from build123d import *

# Parameters (mm, degrees)
SKETCH1_W                                           = 177.8
SKETCH1_H                                           = 150
BOSS_EXTRUDE1_DEPTH                                 = 41.6
SKETCH2_R                                           = 3.683
CUT_EXTRUDE1_DEPTH                                  = 42.6
CUT_EXTRUDE2_DEPTH                                  = 31.6
CBORE_FOR_M4_HEX_SOCKET_HEAD_CAP_SCREW1_D           = 4.5
CBORE_FOR_M4_HEX_SOCKET_HEAD_CAP_SCREW1_CBORE_D     = 8
CBORE_FOR_M4_HEX_SOCKET_HEAD_CAP_SCREW1_CBORE_DEPTH = 32.6
SKETCH9_W                                           = 177.8
SKETCH9_H                                           = 99.2
CUT_EXTRUDE4_DEPTH                                  = 1


with BuildPart() as part:
    # Sketch1 → Boss-Extrude1 (new body)
    with BuildSketch(Plane(origin=(0, 0, 0), x_dir=(1, 0, 0), z_dir=(0, 1, 0))):
        Rectangle(SKETCH1_W, SKETCH1_H)
    extrude(amount=BOSS_EXTRUDE1_DEPTH)

    # Sketch2 → Cut-Extrude1 (cut, through all)
    with BuildSketch(Plane(origin=(0, 41.6, 0), x_dir=(1, 0, 0), z_dir=(0, 1, 0))):
        with Locations(Location((63.5, -63.5, 0), (0, 0, 270))):  # turned: the seam where the file's is
            Circle(SKETCH2_R)
        with Locations(Location((-63.5, -63.5, 0), (0, 0, 270))):  # turned: the seam where the file's is
            Circle(SKETCH2_R)
    cut_extrude1 = extrude(amount=-CUT_EXTRUDE1_DEPTH, mode=Mode.SUBTRACT)

    # Sketch3 → Cut-Extrude2 (cut)
    with BuildSketch(Plane(origin=(0, 41.6, 0), x_dir=(1, 0, 0), z_dir=(0, 1, 0))):
        with BuildLine():
            Line((-74.93, -63.5), (-74.93, -75))
            Line((-74.93, -75), (-52.07, -75))
            Line((-52.07, -75), (-52.07, -63.5))
            ThreePointArc((-52.07, -63.5), (-63.5, -52.07), (-74.93, -63.5))
        make_face()
        with BuildLine():
            Line((52.07, -63.5), (52.07, -75))
            Line((52.07, -75), (74.93, -75))
            Line((74.93, -75), (74.93, -63.5))
            ThreePointArc((74.93, -63.5), (63.5, -52.07), (52.07, -63.5))
        make_face()
    cut_extrude2 = extrude(amount=-CUT_EXTRUDE2_DEPTH, mode=Mode.SUBTRACT)

    # Mirror1: Cut-Extrude1, Cut-Extrude2 across plane
    add(cut_extrude1.mirror(Plane(origin=(0, 0, 0), x_dir=(1, 0, 0), z_dir=(0, 0, -1))), mode=Mode.SUBTRACT)
    add(cut_extrude2.mirror(Plane(origin=(0, 0, 0), x_dir=(1, 0, 0), z_dir=(0, 0, -1))), mode=Mode.SUBTRACT)

    # CBORE for M4 Hex Socket Head Cap Screw1 (through all)
    with Locations(Plane.XZ):
        with Locations((68.9, 0), (-35.089800026, 50), (-35.089800026, -50)):
            CounterBoreHole(CBORE_FOR_M4_HEX_SOCKET_HEAD_CAP_SCREW1_D / 2, CBORE_FOR_M4_HEX_SOCKET_HEAD_CAP_SCREW1_CBORE_D / 2, CBORE_FOR_M4_HEX_SOCKET_HEAD_CAP_SCREW1_CBORE_DEPTH)

    # Sketch9 → Cut-Extrude4 (cut)
    with BuildSketch(Plane.XZ):
        Rectangle(SKETCH9_W, SKETCH9_H)
    extrude(amount=-CUT_EXTRUDE4_DEPTH, mode=Mode.SUBTRACT)


solid = part.part
Can you work these out from the model? Positions are in its coordinate system, mm. A direction names the side the tool comes from. Coordinates: 2 decimals unless noted, no trailing zeros. Loops run counter-clockwise (first coordinate to the right, second up) from the corner with the lowest first, then second, coordinate; pieces in that order, holes last. Notation, with made-up numbers: (88, 69.5) - (104, 69.5) arc R10 ccw to (104, 87.5) - close; hole circle Ø8 at (9, 62). An arc over 180 degrees is marked (long way). Put each result on its own line as item: value. Start each with the question number.
Item 1: Suppose I cut it at A-A (z = 0). Please give me the cut outline in (x, y).
Item 2: If we mould it in two halves opening along Z, with no side actions, what happens to faces 6 (the face through (72.595, 16.579, -1.532)), 7 (the face through (67.15, 5.07, -63.02)), 8 (the face through (63.751, 26.021, 52.073)), 9 (the face through (-52.07, 26, 69))? For each: +Z half, -Z half, draft (parallel to the pull), parting line (faces both ways), or undercut.
Item 3: Which directions (+Z, -Z, +X, -X, +Y, -Y) give clear straight access to the entire face, cutting with the end or side of a thin tool? Please do faces 1 (the face through (-33, 32.6, -52)), 2 (the face through (-59.85, 5.07, -63.02)), 3 (the face through (52.07, 26, -69)), 4 (the face through (52.07, 26, 69)), 5 (the face through (-88.9, 21, 1)).
Item 4: If I drill on line 1 along X through (y, z) = (2.5, -63.5); line 2 along X through (y, z) = (32.5, -59); line 3 along Y through (x, z) = (69, 67.5), over which ranges is the centre line in solid material (lowest first)?
Item 5: Suppose I cut it at B-B (y = 16). Please give me the cut outline in (x, z).
Item 6: Suppose I cut it at C-C (z = 40). Please give me the cut outline in (x, y).
Item 7: For pin 1 (6.5 mm diameter, centred on x = -63.5, z = -63.5, fed in from +Y); pin 2 (4 mm diameter, centred on x = -69.5, z = -35, fed in from -Y); pin 3 (7 mm diameter, centred on x = -35.09, z = 50, fed in from -Y), each with a flat end and sliding along its axis, tell me the tip position at first contact or that it passes through.
Here are the results:
1. outline: (-88.9, 1) - (64.9, 1) - (64.9, 32.6) - (66.65, 32.6) - (66.65, 41.6) - (-88.9, 41.6) - close; (71.15, 32.6) - (72.9, 32.6) - (72.9, 1) - (88.9, 1) - (88.9, 41.6) - (71.15, 41.6) - close
2. face 6: undercut
2. face 7: undercut
2. face 8: +Z half
2. face 9: draft
3. face 1: -Y
3. face 2: +Y, -Y
3. face 3: -Z, +Y
3. face 4: +Z, +Y
3. face 5: +Z, -Z, -X, +Y, -Y
4. line 1: -88.9 to -67.18, -59.82 to 59.82, 67.18 to 88.9
4. line 2: -88.9 to -74.01, -52.99 to 52.99, 74.01 to 88.9
4. line 3: 0 to 10
5. outline: (-88.9, -75) - (-74.93, -75) - (-74.93, -63.5) arc R11.43 cw to (-52.07, -63.5) - (-52.07, -75) - (52.07, -75) - (52.07, -63.5) arc R11.43 cw to (74.93, -63.5) - (74.93, -75) - (88.9, -75) - (88.9, 75) - (74.93, 75) - (74.93, 63.5) arc R11.43 cw to (52.07, 63.5) - (52.07, 75) - (-52.07, 75) - (-52.07, 63.5) arc R11.43 cw to (-74.93, 63.5) - (-74.93, 75) - (-88.9, 75) - close; hole circle Ø8 at (-35.09, -50); hole circle Ø8 at (-35.09, 50); hole circle Ø8 at (68.9, 0)
6. outline: (-88.9, 1) - (88.9, 1) - (88.9, 41.6) - (-88.9, 41.6) - close
7. pin 1: through
7. pin 2: y = 1
7. pin 3: y = 32.6
